Read the model definition and answer for the solid it produces. Units are mm, in the model's axes. A direction names the side the tool comes from. Round coordinates to 2 decimals unless told otherwise and drop trailing zeros. Loops run counter-clockwise (first coordinate to the right, second up) from the corner with the lowest first, then second, coordinate; pieces in that order, holes last. Notation, with made-up numbers: M 28,-28 L 77,-28 A24 cw 77,-6 Z; hole C 76,-33.5 d7. An arc over 180 degrees is marked long. Write each question's results on one line, items separated by ' | '.
```python
from build123d import *

# Parameters (mm, degrees)
SKETCH1_W                       = 48.000000106
SKETCH1_H                       = 198.5
EXTRUDE1_DEPTH                  = 12
SKETCH2_W                       = 3
SKETCH2_H                       = 156.9
EXTRUDE2_DEPTH                  = 13
SKETCH3_R                       = 3.3782
SKETCH3_R_2                     = 0.75
EXTRUDE3_DEPTH                  = 13
SKETCH4_W                       = 12
SKETCH4_H                       = 18
EXTRUDE4_DEPTH                  = 13
FILLET1_R                       = 3
CHAMFER1_SIZE                   = 0.5
EXTRUDE5_DEPTH                  = 20
F_4_40_TAPPED_HOLE1_D           = 2.8448
F_4_40_TAPPED_HOLE2_D           = 2.2606
F_4_40_TAPPED_HOLE2_DEPTH       = 12.6746
F_4_40_TAPPED_HOLE2_CBORE_D     = 2.8448
F_4_40_TAPPED_HOLE2_CBORE_DEPTH = 5.6896
F_4_40_TAPPED_HOLE2_TIP         = 0.679152758
F_1_4_20_TAPPED_HOLE1_D         = 6.35
SKETCH9_R                       = 0.75
EXTRUDE6_DEPTH                  = 8
SKETCH10_R                      = 0.75
EXTRUDE7_DEPTH                  = 8
SKETCH12_R                      = 0.75
EXTRUDE8_DEPTH                  = 8
SKETCH13_R                      = 2.25
CUT_EXTRUDE1_DEPTH              = 13.0000001
SKETCH14_R                      = 0.75
CUT_EXTRUDE2_DEPTH              = 6


with BuildPart() as part:
    # Sketch1 → Extrude1 (new body)
    with BuildSketch(Plane(origin=(0, 0, 0), x_dir=(0, 0, -1), z_dir=(1, 0, 0))):
        with Locations((-24.000000053, 99.25)):
            Rectangle(SKETCH1_W, SKETCH1_H)
    extrude(amount=EXTRUDE1_DEPTH)

    # Sketch2 → Extrude2 (cut, through all)
    with BuildSketch(Plane(origin=(12, 0, 0), x_dir=(0, 0, -1), z_dir=(1, 0, 0))):
        with Locations((-1.5, 120.05)):
            Rectangle(SKETCH2_W, SKETCH2_H)
    extrude(amount=-EXTRUDE2_DEPTH, mode=Mode.SUBTRACT)

    # Sketch3 → Extrude3 (cut, through all)
    with BuildSketch(Plane(origin=(12, 0, 0), x_dir=(0, 0, -1), z_dir=(1, 0, 0))):
        with Locations((-36.000000106, 191.5)):
            Circle(SKETCH3_R)
        with Locations((-11.000000106, 191.5)):
            Circle(SKETCH3_R)
        with Locations((-38.000000106, 7)):
            Circle(SKETCH3_R)
        with Locations((-10.000000106, 7)):
            Circle(SKETCH3_R)
        with Locations((-23.000000106, 56.6)):
            Circle(SKETCH3_R_2)
        with Locations((-23.000000106, 121.6)):
            Circle(SKETCH3_R_2)
    extrude(amount=-EXTRUDE3_DEPTH, mode=Mode.SUBTRACT)

    # Sketch4 → Extrude4 (cut, through all)
    with BuildSketch(Plane(origin=(12, 0, 0), x_dir=(0, 0, -1), z_dir=(1, 0, 0))):
        with Locations((-29.000000106, 91.6)):
            Rectangle(SKETCH4_W, SKETCH4_H)
    extrude(amount=-EXTRUDE4_DEPTH, mode=Mode.SUBTRACT)

    # Fillet1
    fillet1_edges = [part.edges().sort_by_distance(p)[0] for p in [
        (6, 82.6, 35.000000106),
        (6, 100.6, 35.000000106),
        (6, 100.6, 23.000000106),
        (6, 82.6, 23.000000106),
    ]]
    fillet(fillet1_edges, radius=FILLET1_R)

    # Chamfer1
    chamfer1_edges = [part.edges().sort_by_distance(p)[0] for p in [
        (12, 91.6, 35.000000106),
        (0, 91.6, 35.000000106),
        (12, 100.6, 29.000000106),
        (0, 100.6, 29.000000106),
        (12, 91.6, 23.000000106),
        (0, 91.6, 23.000000106),
        (12, 82.6, 29.000000106),
        (0, 82.6, 29.000000106),
        (12, 99.721320344, 34.12132045),
        (0, 99.721320344, 34.12132045),
        (12, 99.721320344, 23.878679762),
        (0, 99.721320344, 23.878679762),
        (12, 83.478679656, 23.878679762),
        (0, 83.478679656, 23.878679762),
        (12, 83.478679656, 34.12132045),
        (0, 83.478679656, 34.12132045),
    ]]
    chamfer(chamfer1_edges, length=CHAMFER1_SIZE)

    # Sketch5 → Extrude5 (cut)
    with BuildSketch(Plane.XZ):
        Polygon((0, 0), (4, 0), (0, 4), align=None)
    extrude5 = extrude(amount=-EXTRUDE5_DEPTH, mode=Mode.SUBTRACT)

    # Mirror1: Extrude5 across plane
    add(extrude5.mirror(Plane(origin=(6, 0, 0), x_dir=(0, 0, 1), z_dir=(1, 0, 0))), mode=Mode.SUBTRACT)

    # #4-40 Tapped Hole1 (through all)
    with Locations(Plane(origin=(12, 106.6, 9.35), x_dir=(0, 0, 1), z_dir=(1, 0, 0))):
        with Locations((0, 0), (0, 30)):
            Hole(F_4_40_TAPPED_HOLE1_D / 2)

    # #4-40 Tapped Hole2
    with Locations(Plane(origin=(6, 96.6, 48.000000106), x_dir=(1, 0, 0), z_dir=(0, 0, 1))):
        with Locations((0, 0), (0, -10)):
            CounterBoreHole(F_4_40_TAPPED_HOLE2_D / 2, F_4_40_TAPPED_HOLE2_CBORE_D / 2, F_4_40_TAPPED_HOLE2_CBORE_DEPTH, depth=F_4_40_TAPPED_HOLE2_DEPTH)
            with Locations((0, 0, -(F_4_40_TAPPED_HOLE2_DEPTH + F_4_40_TAPPED_HOLE2_TIP / 2))):  # 118° drill point
                Cone(0, F_4_40_TAPPED_HOLE2_D / 2, F_4_40_TAPPED_HOLE2_TIP, mode=Mode.SUBTRACT)

    # 1/4-20 Tapped Hole1 (through all)
    with Locations(Plane(origin=(6, 121.6, 48.000000106), x_dir=(1, 0, 0), z_dir=(0, 0, 1))):
        with Locations((0, 0), (0, -65)):
            Hole(F_1_4_20_TAPPED_HOLE1_D / 2)

    # Sketch9 → Extrude6 (cut)
    with BuildSketch(Plane.XY.offset(48.000000106)):
        with Locations((6, 7)):
            Circle(SKETCH9_R)
        with Locations((6, 191.5)):
            Circle(SKETCH9_R)
    extrude(amount=-EXTRUDE6_DEPTH, mode=Mode.SUBTRACT)

    # Sketch10 → Extrude7 (cut)
    with BuildSketch(Plane(origin=(0, 0, 3), x_dir=(-1, 0, 0), z_dir=(0, 0, -1))):
        with Locations(Location((-6, 191.5, 0), (0, 0, 180))):  # turned: the seam where the file's is
            Circle(SKETCH10_R)
    extrude(amount=-EXTRUDE7_DEPTH, mode=Mode.SUBTRACT)

    # Sketch12 → Extrude8 (cut)
    with BuildSketch(Plane(origin=(0, 0, 0), x_dir=(-1, 0, 0), z_dir=(0, 0, -1))):
        with Locations(Location((-6, 7, 0), (0, 0, 180))):  # turned: the seam where the file's is
            Circle(SKETCH12_R)
    extrude(amount=-EXTRUDE8_DEPTH, mode=Mode.SUBTRACT)

    # Sketch13 → Cut-Extrude1 (cut, through all)
    with BuildSketch(Plane(origin=(12, 0, 0), x_dir=(0, 0, -1), z_dir=(1, 0, 0))):
        with Locations((-42.000000106, 162)):
            Circle(SKETCH13_R)
        with Locations((-42.000000106, 150)):
            Circle(SKETCH13_R)
    extrude(amount=-CUT_EXTRUDE1_DEPTH, mode=Mode.SUBTRACT)

    # Sketch14 → Cut-Extrude2 (cut)
    with BuildSketch(Plane.XY.offset(48.000000106)):
        with Locations((6, 162)):
            Circle(SKETCH14_R)
        with Locations((6, 150)):
            Circle(SKETCH14_R)
    extrude(amount=-CUT_EXTRUDE2_DEPTH, mode=Mode.SUBTRACT)


solid = part.part
```
1. Find section A-A, the plane z = 37.5. Give the vertices of the cut face in (x, y) (3 decimals).
Completed:
outline: M 0,0 L 12,0 L 12,3.659 L 0,3.659 Z; M 0,10.341 L 12,10.341 L 12,188.473 L 0,188.473 Z; M 0,194.527 L 12,194.527 L 12,198.5 L 0,198.5 Z; hole C 6,56.6 d6.35; hole C 6,121.6 d6.35; hole C 6,86.6 d2.261; hole C 6,96.6 d2.261
2. Which of the six approach directions +Z, -Z, +X, -X, +Y, -Y give full straight-line access (tool end or side, diameter ignored) to faces 5 (the face through (9, 119, 3)), 6 (the face through (11.642, 99.797, 34.246)), 7 (the face through (0.365, 99.841, 23.807))?
Completed:
face 5: -Z, +X, -X, +Y | face 6: +X | face 7: -X
3. Given P1, Ø0.9, axis at x = 6, y = 150, coming from the -Z side, flat-ended and moving along its own axis, determine where the tip first touches the part or whether it passes through.
Completed:
P1: stops at z = 3
4. Find section B-B, the plane y = 158. Give the vertices of the cut face in (x, z).
Completed:
outline: M 0,3 L 12,3 L 12,48 L 0,48 Z
5. Find the intervals of material crossed by L1, parallel to Y at x = 8.5, z = 25.5; L2, parallel to Y at x = 8, z = 42; L3, parallel to Z at x = 10.15, y = 121.6, in increasing order.
Completed:
L1: y = 0 to 54.64, 58.56 to 82.64, 100.56 to 119.64, 123.56 to 198.5 | L2: y = 0 to 54.13, 59.07 to 119.13, 124.07 to 147.75, 152.25 to 159.75, 164.25 to 198.5 | L3: z = 3 to 22.25, 23.75 to 48
6. Determine the mould class of faces 1 (the face through (4.293, 59.277, 25.185)), 2 (the face through (11.642, 83.403, 23.754)), 3 (the face through (11.642, 83.354, 34.197)), 4 (the face through (2, 10, 2)) for opening direction Z: released by +Z, released by -Z, zero draft, split by the parting line, or undercut.
Completed:
face 1: zero draft | face 2: undercut | face 3: undercut | face 4: released by -Z
